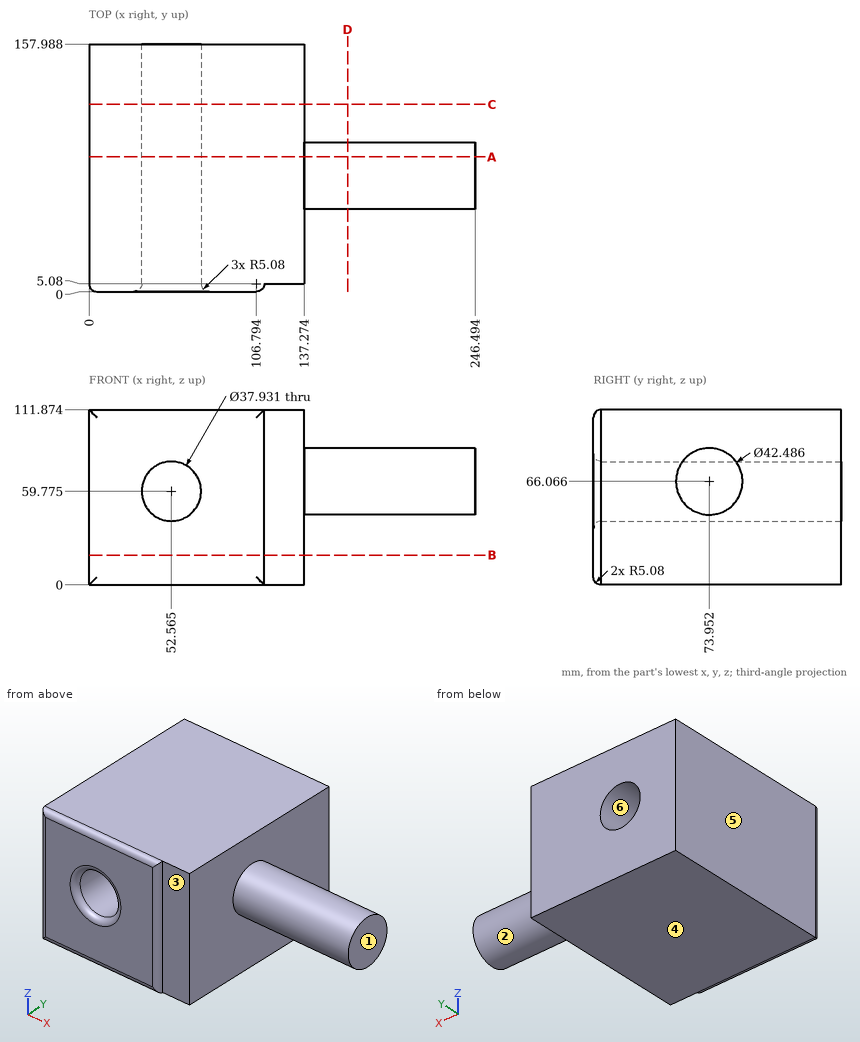
For this review, use the dimensioned drawing (mm, ordinates from the lowest corner) and the shaded views. A direction names the side the tool comes from. Round coordinates to 2 decimals unless told otherwise and drop trailing zeros. Order: outer loops, then holes, each group sorted by start corner. A loop starts at its lowest first (then second) coordinate and runs counter-clockwise, first axis right, second up. Notation, with made-up numbers: (-35, 12) -> (7, 12) arc R17 ccw to (7, 43) -> close; hole circle Ø5 at (63.25, 69). An arc over 180 degrees is marked (long way). Use CSV: the item, a comma, the result in double quotes. Start each with the question number.
(1) Consider section B-B on z = 19. Write out the cut boundary in (x, y) (1 decimal).
(2) Consider section C-C on y = 119.5. Write out the cut boundary in (x, z) (1 decimal), and give its area (3 significant figures).
(3) Consider section D-D on x = 165. Write out the cut boundary in (y, z) (1 decimal), and give its area (3 significant figures).
(4) Mouldability with a two-part tool opening along Z and no side actions: class the marked faces 4, 5 and 6 as pulls with the +Z half, pulls with the -Z half, needs draft (parallel to the pull), parting line crosses it, or undercut.
(5) Wall thickness on probe 1 along Y at (x, z) = (107.5, 42); probe 2 along X at (y, z) = (18.5, 36.5) (1 decimal); probe 3 along X at (y, z) = (53.5, 70) (1 decimal): over which ranges is each line inside the solid? List them lowest first. Write a range as from..to.
(6) Tool access review of the marked faces 1, 2 and 3: name each direction out of +Z, -Z, +X, -X, +Y, -Y from which nothing blocks a thin tool from reaching the whole face with its end or side.
(7) Insertion check: pin 1 (12.5 mm diameter, centred on x = 127.5, z = 65.5, fed in from -Y); pin 2 (1 mm diameter, centred on y = 106, z = 78, fed in from +X). Each pin has a flat end and moves straight along its axis. Give the tip position at first contact, or say it passes through.
(8) Consider section A-A on y = 86. Write out the cut boundary in (x, z) (1 decimal), and give its area (4 significant figures).
Responses:
1,outline,"(0, 5.1) arc R5.1 ccw to (5.1, 0) -> (106.8, 0) arc R5.1 ccw to (111.9, 5.1) -> (137.3, 5.1) -> (137.3, 158) -> (0, 158) -> close"
2,outline,"(0, 0) -> (137.3, 0) -> (137.3, 111.9) -> (0, 111.9) -> close; hole circle Ø37.9 at (52.6, 59.8)"
2,area,"14,200 mm²"
3,outline,"circle Ø42.5 at (74, 66.1)"
3,area,"1,420 mm²"
4,face 4,"pulls with the -Z half"
4,face 5,"needs draft"
4,face 6,"undercut"
5,probe 1,"0.05..157.99"
5,probe 2,"0..137.3"
5,probe 3,"0..36.6, 68.5..246.5"
6,face 1,"+Z, -Z, +X, +Y, -Y"
6,face 2,"+X"
6,face 3,"+Z, -Z, +X, -Y"
7,pin 1,"y = 5.08"
7,pin 2,"x = 137.27"
8,outline,"(0, 0) -> (137.3, 0) -> (137.3, 48.6) -> (246.5, 48.6) -> (246.5, 83.6) -> (137.3, 83.6) -> (137.3, 111.9) -> (0, 111.9) -> close; hole circle Ø37.9 at (52.6, 59.8)"
8,area,"18,050 mm²"
